Autodesk Inventor part; units mm, degrees
ref_plane "YZ Plane" through (0, 0, 0) normal (1, 0, 0) x (0, 1, 0)
ref_plane "XZ Plane" through (0, 0, 0) normal (0, 1, 0) x (-1, 0, 0)
ref_plane "XY Plane" through (0, 0, 0) normal (0, 0, 1) x (1, 0, 0)
sketch "Sketch1" plane through (0, 0, 0) normal (0, 1, 0) x (-1, 0, 0)
  line L0 (0, 0) -> (9, 0)
  line L1 (9, 0) -> (9, -25)
  line L2 (9, -25) -> (0, -25)
  line L3 (0, -25) -> (0, 0)
  circle A0 centre (4.5, -5) radius 1.7
  circle A1 centre (4.5, -20) radius 1.7
  line L4 (4.5, 0) -> (4.5, -25) construction
  line L5 (9, -12.5) -> (0, -12.5) construction
  dimension "d0" = 9
  dimension "d1" = 3.4
  dimension "d2" = 3.4
  dimension "d3" = 7.5
  dimension "d4" = 7.5
  dimension "d5" = 25
extrude "Extrusion1" add sketch "Sketch1" along normal blind 4.2
sketch "Sketch2" plane through (0, 0, 0) normal (1, 0, 0) x (0, 0, -1)
  line L0 (0, 0) -> (25, 0) construction
  line L1 (12.5, 0) -> (12.5, 1.1571) construction
  line L2 (12.5, 1.1571) -> (11.3429, 0)
  line L3 (12.5, 1.1571) -> (13.6571, 0)
  line L4 (9.1461, 0) -> (13.6571, 0)
  circle A0 centre (12.5, 0.45) radius 0.5
  point P0 (11.3429, 0)
  dimension "d8" = 45
  dimension "d10" = 45
  dimension "d14" = 1
  dimension "d15" = 0.45
extrude "Extrusion2" cut sketch "Sketch2" against normal through all contours L3 A0 L2 | A0 L4 L2 | A0 L4 | L3 L4 A0 picked at (12.3997, 0.4044)
equation "\"d1\" = d2"
equation "\"d4\" = d3"
equation "\"d10\" = d8"
properties part number "suction_electrode_holder"
Can you work these out from the model? Positions are in its coordinate system, mm. A direction names the side the tool comes from. Round coordinates to 2 decimals unless told otherwise and drop trailing zeros. Loops run counter-clockwise (first coordinate to the right, second up) from the corner with the lowest first, then second, coordinate; pieces in that order, holes last. Notation, with made-up numbers: (-3, -10.5) -> (28, -10.5) arc R24 ccw to (28, 12.5) -> close; hole circle Ø2 at (3.25, -6). An arc over 180 degrees is marked (long way). One line per item, written item: value. Start each with the question number.
1. If we section it at C-C, the plane x = -4.5: Write out the boundary of the cut face in (y, z), then the cut area to 3 significant figures.
2. If I drill on probe 1 along Z at (x, y) = (-4.5, 2.7); probe 2 along Z at (x, y) = (-5, 0.75); probe 3 along X at (y, z) = (3.5, -21), over which ranges is the centre line in solid material (lowest first)?
3. If we section it at B-B, the plane y = 2.5: Write out the boundary of the cut face in (x, z), then the cut area to 3 significant figures.
4. If we section it at A-A, the plane z = -20: Write out the boundary of the cut face in (x, y), then the cut area to 3 significant figures.
5. For faces 5 (the flat face through (-9, 2, -12)), 6 (the flat face through (-4.437, 0.587, -13.07)), which set-ups out of +Z, -Z, +X, -X, +Y, -Y let a thin tool reach every point of the face, with its end or its side?
6. If we mould it in two halves opening along Z, with no side actions, what happens to faces 1 (the flat face through (-4, 0, -7)), 2 (the flat face through (-4, 2, 0)), 3 (the flat face through (-4.437, 0.587, -11.93)), 4 (the cylindrical face through (-5.3, 2.1, -3.5))? For each: pulls with the +Z half, pulls with the -Z half, needs draft (parallel to the pull), parting line crosses it, or undercut.
7. For pin 1 (2 mm diameter, centred on x = -4.5, z = -20, fed in from +Y), with a flat end and sliding along its axis, tell me the tip position at first contact or that it passes through.
Calculated:
1. outline: (0, -25) -> (4.2, -25) -> (4.2, -21.7) -> (0, -21.7) -> close; (0, -18.3) -> (4.2, -18.3) -> (4.2, -6.7) -> (0, -6.7) -> (0, -11.34) -> (1.16, -12.5) -> (0, -13.66) -> close; (0, -3.3) -> (4.2, -3.3) -> (4.2, 0) -> (0, 0) -> close
1. area: 75.1 mm²
2. probe 1: z = -25 to -21.7, -18.3 to -6.7, -3.3 to 0
2. probe 2: z = -25 to -21.62, -18.38 to -12.91, -12.09 to -6.62, -3.38 to 0
2. probe 3: x = -9 to -5.87, -3.13 to 0
3. outline: (-9, -25) -> (0, -25) -> (0, 0) -> (-9, 0) -> close; hole circle Ø3.4 at (-4.5, -20); hole circle Ø3.4 at (-4.5, -5)
3. area: 207 mm²
4. outline: (-9, 0) -> (-6.2, 0) -> (-6.2, 4.2) -> (-9, 4.2) -> close; (-2.8, 0) -> (0, 0) -> (0, 4.2) -> (-2.8, 4.2) -> close
4. area: 23.5 mm²
5. face 5: +Z, -Z, -X, +Y, -Y
5. face 6: +X, -X, -Y
6. face 1: needs draft
6. face 2: pulls with the +Z half
6. face 3: undercut
6. face 4: undercut
7. pin 1: passes through
